from build123d import *

# Parameters (mm, degrees)
SKETCH_1_W          = 24
SKETCH_1_H          = 24
EXTRUDE_1_DEPTH     = 42
SKETCH_3_R          = 10.5
CUT_EXTRUDE_1_DEPTH = 20
SKETCH_4_W          = 17
SKETCH_4_H          = 17
CUT_EXTRUDE_2_DEPTH = 20
SKETCH_5_W          = 15
SKETCH_5_H          = 15
CUT_EXTRUDE_5_DEPTH = 50.839743178
SKETCH_6_W          = 7
SKETCH_6_H          = 7
SKETCH_6_R          = 1.5
EXTRUDE_2_DEPTH     = 2


with BuildPart() as part:
    # Эскиз1 → Бобышка-Вытянуть1 (new body)
    with BuildSketch(Plane.XY):
        Rectangle(SKETCH_1_W, SKETCH_1_H)
    extrude(amount=EXTRUDE_1_DEPTH)

    # Эскиз3 → Вырез-Вытянуть1 (cut)
    with BuildSketch(Plane.XY.offset(42)):
        Circle(SKETCH_3_R)
    extrude(amount=-CUT_EXTRUDE_1_DEPTH, mode=Mode.SUBTRACT)

    # Эскиз4 → Вырез-Вытянуть2 (cut)
    with BuildSketch(Plane.XY.offset(22)):
        Rectangle(SKETCH_4_W, SKETCH_4_H)
    extrude(amount=-CUT_EXTRUDE_2_DEPTH, mode=Mode.SUBTRACT)

    # Эскиз5 → Вырез-Вытянуть5 (cut, through all)
    with BuildSketch(Plane(origin=(12, 0, 0), x_dir=(0, 0, -1), z_dir=(1, 0, 0))):
        with Locations((-9.5, -1)):
            Rectangle(SKETCH_5_W, SKETCH_5_H)
    extrude(amount=-CUT_EXTRUDE_5_DEPTH, mode=Mode.SUBTRACT)

    # Эскиз6 → Бобышка-Вытянуть2 (add)
    # profile 1 of 2: a face of its own
    with BuildSketch(Plane(origin=(12, 0, 0), x_dir=(0, 0, -1), z_dir=(1, 0, 0))):
        with Locations((-9.5, 15.5)):
            Rectangle(SKETCH_6_W, SKETCH_6_H)
        with Locations((-9.5, 15.5)):
            Circle(SKETCH_6_R, mode=Mode.SUBTRACT)
    # profile 2 of 2: a face of its own
    with BuildSketch(Plane(origin=(12, 0, 0), x_dir=(0, 0, -1), z_dir=(1, 0, 0))):
        with Locations((-9.5, -15.5)):
            Rectangle(SKETCH_6_W, SKETCH_6_H)
        with Locations((-9.5, -15.5)):
            Circle(SKETCH_6_R, mode=Mode.SUBTRACT)
    extrude(amount=-EXTRUDE_2_DEPTH)


solid = part.part
Could you check a few things on this model? Use its own coordinates, in mm. A direction names the side the tool comes from. Round coordinates to 2 decimals unless told otherwise and drop trailing zeros. Write each loop counter-clockwise with the first axis right and the second up, starting at its lowest first coordinate (ties: lowest second). Pieces come first, ordered by that corner, then holes. Notation, with made-up numbers: (77.5, 0.25) - (97.5, 0.25) arc R21 cw to (97.5, 8.25) - close; hole circle Ø10 at (-27, 49.25). An arc over 180 degrees is marked (long way). Use a Markdown table: item, result.
Q1. For pin 1 (1 mm diameter, centred on x = -9.5, y = 0.5, fed in from +Z); pin 2 (6 mm diameter, centred on x = -5.5, z = 14, fed in from +Y); pin 3 (1.6 mm diameter, centred on x = 11, y = -15, fed in from -Z), each with a flat end and sliding along its axis, tell me the tip position at first contact or that it passes through.
Output values:
| item | result |
|---|---|
| pin 1 | z = 22 |
| pin 2 | y = 12 |
| pin 3 | z = 6 |
Q2. I want a section at A-A (y = -15.5). List the corners of the cut face in (x, z) for me, plus the area to 3 significant figures.
Output values:
| item | result |
|---|---|
| outline | (10, 6) - (12, 6) - (12, 8) - (10, 8) - close; (10, 11) - (12, 11) - (12, 13) - (10, 13) - close |
| area | 8.00 mm2 |
Q3. Thinking about a two-plate mould opening in Y: for faces 1 (the flat face through (11, 19, 10)), 2 (the flat face through (12, 0, 21)), 3 (the flat face through (0, 0, 2)), which applies, released by +Y, released by -Y, zero draft, split by the parting line, or undercut?
Output values:
| item | result |
|---|---|
| face 1 | released by +Y |
| face 2 | zero draft |
| face 3 | undercut |
Q4. For faces 4 (the flat face through (11, -16, 13)), 5 (the flat face through (10, -14.7, 11.1)), 6 (the flat face through (8, -8, 22)), 7 (the flat face through (-10, 6.5, 10)), which set-ups out of +Z, -Z, +X, -X, +Y, -Y let a thin tool reach every point of the face, with its end or its side?
Output values:
| item | result |
|---|---|
| face 4 | +Z, +X, -X, -Y |
| face 5 | +Z, -Z, -X, -Y |
| face 6 | none |
| face 7 | +X, -X |
Q5. I want a section at B-B (z = 13.5). List the corners of the cut face in (x, y) for me, plus the area to 3 significant figures.
Output values:
| item | result |
|---|---|
| outline | (-12, -12) - (12, -12) - (12, -8.5) - (-12, -8.5) - close; (-12, 6.5) - (-8.5, 6.5) - (-8.5, 8.5) - (8.5, 8.5) - (8.5, 6.5) - (12, 6.5) - (12, 12) - (-12, 12) - close |
| area | 182 mm2 |
Q6. Please list where these lines run through material, in increasing order: L1, parallel to Y at x = 10.8, z = 9.5; L2, parallel to Y at x = -2, z = 7.5; L3, parallel to X at y = 0.5, z = 39.5.
Output values:
| item | result |
|---|---|
| L1 | -19 to -17, -14 to -8.5, 6.5 to 14, 17 to 19 |
| L2 | -12 to -8.5, 8.5 to 12 |
| L3 | -12 to -10.49, 10.49 to 12 |
Q7. I want a section at C-C (x = 0). List the corners of the cut face in (y, z) for me, plus the area to 3 significant figures.
Output values:
| item | result |
|---|---|
| outline | (-12, 0) - (12, 0) - (12, 42) - (10.5, 42) - (10.5, 22) - (8.5, 22) - (8.5, 2) - (-8.5, 2) - (-8.5, 22) - (-10.5, 22) - (-10.5, 42) - (-12, 42) - close |
| area | 248 mm2 |
Q8. I want a section at D-D (z = 31). List the corners of the cut face in (x, y) for me.
Output values:
| item | result |
|---|---|
| outline | (-12, -12) - (12, -12) - (12, 12) - (-12, 12) - close; hole circle Ø21 at (0, 0) |
